Input: part model. Units: mm. Frame: model coordinates. A direction names the side the tool comes from. Round coordinates to 2 decimals unless told otherwise and drop trailing zeros. Order: outer loops, then holes, each group sorted by start corner. A loop starts at its lowest first (then second) coordinate and runs counter-clockwise, first axis right, second up. Notation, with made-up numbers: (-28.5, -13.75) -> (3.5, -13.75) arc R19 cw to (3.5, 9.25) -> close; hole circle Ø6 at (47.25, 73). An arc over 180 degrees is marked (long way). Use a Markdown table: item, result.
from build123d import *

# Parameters (mm, degrees)
ESQUISSE1_W             = 25
ESQUISSE1_H             = 40
BOSS_EXTRU_1_DEPTH      = 5
ESQUISSE2_R             = 1.625
ENL_V_MAT_EXTRU_1_DEPTH = 6
ESQUISSE3_W             = 15
ESQUISSE3_H             = 40
BOSS_EXTRU_2_DEPTH      = 25
ESQUISSE4_W             = 12.4
ESQUISSE4_H             = 23.4
ENL_V_MAT_EXTRU_2_DEPTH = 14
ESQUISSE5_W             = 5
ESQUISSE5_H             = 4
ENL_V_MAT_EXTRU_3_DEPTH = 26


with BuildPart() as part:
    # Esquisse1 → Boss.-Extru.1 (new body)
    with BuildSketch(Plane.XY):
        with Locations((12.5, -20)):
            Rectangle(ESQUISSE1_W, ESQUISSE1_H)
    extrude(amount=BOSS_EXTRU_1_DEPTH)

    # Esquisse2 → Enlèv. mat.-Extru.1 (cut, through all)
    with BuildSketch(Plane.XY.offset(5)):
        with Locations((5, -5)):
            Circle(ESQUISSE2_R)
        with Locations((5, -35)):
            Circle(ESQUISSE2_R)
    extrude(amount=-ENL_V_MAT_EXTRU_1_DEPTH, mode=Mode.SUBTRACT)

    # Esquisse3 → Boss.-Extru.2 (add)
    with BuildSketch(Plane.XY.offset(5)):
        with Locations((17.5, -20)):
            Rectangle(ESQUISSE3_W, ESQUISSE3_H)
    extrude(amount=BOSS_EXTRU_2_DEPTH)

    # Esquisse4 → Enlèv. mat.-Extru.2 (cut)
    with BuildSketch(Plane(origin=(25, 0, 0), x_dir=(0, 0, -1), z_dir=(1, 0, 0))):
        with Locations((-20.8, -14.7)):
            Rectangle(ESQUISSE4_W, ESQUISSE4_H)
    extrude(amount=-ENL_V_MAT_EXTRU_2_DEPTH, mode=Mode.SUBTRACT)

    # Esquisse5 → Enlèv. mat.-Extru.3 (cut, through all)
    with BuildSketch(Plane(origin=(25, 0, 0), x_dir=(0, 0, -1), z_dir=(1, 0, 0))):
        with Locations((-20.8, -3)):
            Rectangle(ESQUISSE5_W, ESQUISSE5_H)
    extrude(amount=-ENL_V_MAT_EXTRU_3_DEPTH, mode=Mode.SUBTRACT)


solid = part.part
1) Ray query, probe 1 along Y at (x, z) = (5, 1.8) (3 decimals); probe 2 along Z at (x, y) = (23.25, -25); probe 3 along Y at (x, z) = (21, 17). Return the intervals inside material, ascending.
Answer key:
| item | result |
|---|---|
| probe 1 | y = -40 to -36.625, -33.375 to -6.625, -3.375 to 0 |
| probe 2 | z = 0 to 14.6, 27 to 30 |
| probe 3 | y = -40 to -26.4, -3 to 0 |
2) Set-up query: faces 1 (the face through (18, -1, 21)), 2 (the face through (10, -20, 17)), 3 (the face through (18, -15, 27)), 4 (the face through (3.802, -3.902, 2.535)). Return all of +Z, -Z, +X, -X, +Y, -Y with unobstructed straight access to the full face (end or side cutting, diameter ignored); none if empty.
Answer key:
| item | result |
|---|---|
| face 1 | +X, -X |
| face 2 | +Z, -X, +Y, -Y |
| face 3 | +X |
| face 4 | +Z, -Z |
3) Contact query for flat-ended pins moving along their axis: P1, Ø6, axis at y = -10.5, z = 19, coming from the +X side; P2, Ø2, axis at x = 8.5, z = 21.5, coming from the -Y side; P3, Ø3, axis at x = 3, y = -22, coming from the +Z side. Output: stop coordinate, or through.
Answer key:
| item | result |
|---|---|
| P1 | stops at x = 11 |
| P2 | passes through |
| P3 | stops at z = 5 |
4) Cut plane D-D on z = 4.25. Return loops of the section in (x, y) (3 decimals).
Answer key:
| item | result |
|---|---|
| outline | (0, -40) -> (25, -40) -> (25, 0) -> (0, 0) -> close; hole circle Ø3.25 at (5, -35); hole circle Ø3.25 at (5, -5) |
5) Draft query along Z for faces 5 (the face through (25, -20, 11)), 6 (the face through (5, -20, 5)), 7 (the face through (18, -3, 16)). Return one class per face: released by +Z, released by -Z, zero draft, split by the parting line, or undercut.
Answer key:
| item | result |
|---|---|
| face 5 | zero draft |
| face 6 | released by +Z |
| face 7 | undercut |
6) Cut plane A-A on x = 5. Return loops of the section in (y, z) (3 decimals).
Answer key:
| item | result |
|---|---|
| outline | (-40, 0) -> (-36.625, 0) -> (-36.625, 5) -> (-40, 5) -> close; (-33.375, 0) -> (-6.625, 0) -> (-6.625, 5) -> (-33.375, 5) -> close; (-3.375, 0) -> (0, 0) -> (0, 5) -> (-3.375, 5) -> close |
7) Cut plane B-B on y = -2.5. Return loops of the section in (x, z).
Answer key:
| item | result |
|---|---|
| outline | (0, 0) -> (25, 0) -> (25, 18.3) -> (10, 18.3) -> (10, 5) -> (0, 5) -> close; (10, 23.3) -> (25, 23.3) -> (25, 30) -> (10, 30) -> close |
8) Cut plane C-C on x = 18.5. Return loops of the section in (y, z).
Answer key:
| item | result |
|---|---|
| outline | (-40, 0) -> (0, 0) -> (0, 30) -> (-40, 30) -> close; hole (-26.4, 14.6) -> (-3, 14.6) -> (-3, 18.3) -> (-1, 18.3) -> (-1, 23.3) -> (-3, 23.3) -> (-3, 27) -> (-26.4, 27) -> close |
